Check sheet for the modelled part. Datum: model origin and axes. Units: mm. Face numbers are marked on the shaded views. Give positions to 0.01 mm unless a question says otherwise; leave off trailing zeros. Write each loop counter-clockwise with the first axis right and the second up, starting at its lowest first coordinate (ties: lowest second). Pieces come first, ordered by that corner, then holes. Notation, with made-up numbers: M 59,76 L 77,76 A21 ccw 77,84 Z; hole C 4.5,19 d1. An arc over 180 degrees is marked long. Use CSV: the item, a comma, the result in double quotes. Start each with the question number.
1. Cross-section at A-A, the plane x = -2.25. Enter the section's corners in (y, z).
2. Cross-section at D-D, the plane x = -1. Enter the section's corners in (y, z), and give its area (3 significant figures).
3. Mould release check, pull along Z, two halves, no side actions. Record for the marked faces 1, 2 and 3: +Z half, -Z half, draft (parallel to the pull), parting line (faces both ways), or undercut.
4. Depth check by flat-ended pin: P1, Ø4, axis at x = 3, y = 2, coming from the -Z side. Enter the tip coordinate at first touch or a pass-through.
5. Cross-section at B-B, the plane y = 3.5. Enter the section's corners in (x, z).
6. Cross-section at C-C, the plane z = 0.8. Enter the section's corners in (x, y), and give its area (3 significant figures).
7. Scan lines: line 1 (Z direction, x = -5.5, y = -2.75); line 2 (X direction, y = -4, z = 1.2); line 3 (X direction, y = -3, z = 0.9). Record each from-to range of solid material in increasing order.
Autodesk Inventor part; units mm, degrees
ref_plane "YZ Plane" through (0, 0, 0) normal (1, 0, 0) x (0, 1, 0)
ref_plane "XZ Plane" through (0, 0, 0) normal (0, 1, 0) x (-1, 0, 0)
ref_plane "XY Plane" through (0, 0, 0) normal (0, 0, 1) x (1, 0, 0)
sketch "Náčrt1" plane through (0, 0, 0) normal (0, 0, 1) x (1, 0, 0)
  line L0 (0, 8.68) -> (0, -8.68)
  line L1 (-8.68, 0) -> (8.68, 0)
  circle A0 centre (0, 0) radius 6.2
  dimension "d0" = 12.4
extrude "Vysunutí1" add sketch "Náčrt1" along normal blind 1
sketch "Náčrt2" plane through (0, 0, 1) normal (0, 0, 1) x (1, 0, 0)
  line L0 (-8.68, 0) -> (8.68, 0)
  line L1 (0, 8.68) -> (0, -8.68)
  line L2 (0, 1.5556) -> (-2.7577, 4.3134)
  line L3 (-2.7577, 4.3134) -> (-4.3134, 2.7577)
  line L4 (-4.3134, 2.7577) -> (-1.5556, 0)
  line L5 (0, 0) -> (-4.3841, 4.3841)
  circle A0 centre (0, 0) radius 6.2
  line L6 (0, 0) -> (6.2, 0) construction
  line L7 (-4.3134, -2.7577) -> (-2.7577, -4.3134)
  line L8 (-1.5556, 0) -> (-4.3134, -2.7577)
  line L9 (-2.7577, -4.3134) -> (0, -1.5556)
  line L10 (2.7577, -4.3134) -> (4.3134, -2.7577)
  line L11 (0, -1.5556) -> (2.7577, -4.3134)
  line L12 (4.3134, -2.7577) -> (1.5556, 0)
  line L13 (4.3134, 2.7577) -> (2.7577, 4.3134)
  line L14 (1.5556, 0) -> (4.3134, 2.7577)
  line L15 (2.7577, 4.3134) -> (0, 1.5556)
  point P0 (-1.5556, 0)
  point P1 (0, -1.5556)
  point P2 (1.5556, 0)
  dimension "d3" = 2.2
  dimension "d4" = 5
  dimension "d5" = 135
  dimension "d8" = 360
extrude "Vysunutí2" add sketch "Náčrt2" along normal blind 0.4 contours L4 L3 L5 L0 | L0 L1 L9 L7 L8 | L1 L15 L13 L14 L0 | L5 L3 L2 L1 | L0 L12 L10 L11 L1
properties part number "button_plate_cross"
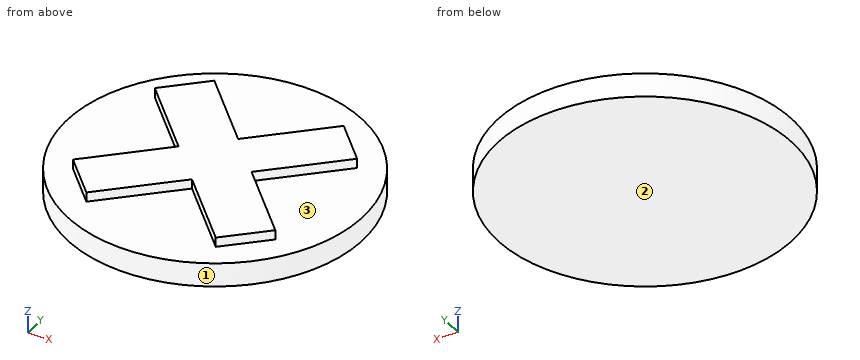
Worked answers:
1,outline,"M -5.78,0 L 5.78,0 L 5.78,1 L 3.81,1 L 3.81,1.4 L 0.69,1.4 L 0.69,1 L -0.69,1 L -0.69,1.4 L -3.81,1.4 L -3.81,1 L -5.78,1 Z"
2,outline,"M -6.12,0 L 6.12,0 L 6.12,1 L 2.56,1 L 2.56,1.4 L -2.56,1.4 L -2.56,1 L -6.12,1 Z"
2,area,"14.3 mm^2"
3,face 1,"draft"
3,face 2,"-Z half"
3,face 3,"+Z half"
4,P1,"stops at z = 0"
5,outline,"M -5.12,0 L 5.12,0 L 5.12,1 L 3.57,1 L 3.57,1.4 L 1.94,1.4 L 1.94,1 L -1.94,1 L -1.94,1.4 L -3.57,1.4 L -3.57,1 L -5.12,1 Z"
6,outline,"C 0,0 d12.4"
6,area,"121 mm^2"
7,line 1,"z = 0 to 1"
7,line 2,"x = -3.07 to -2.44, 2.44 to 3.07"
7,line 3,"x = -5.43 to 5.43"
